Source: three-view drawing plus pictorial views. Frame: mm from the lowest corner of the part. A direction names the side the tool comes from. Coordinates: 2 decimals unless noted, no trailing zeros. Loops run counter-clockwise (first coordinate to the right, second up) from the corner with the lowest first, then second, coordinate; pieces in that order, holes last. Notation, with made-up numbers: M 34.5,78.5 L 60.5,78.5 A22 ccw 60.5,117.5 Z; hole C 28,-26 d6. An arc over 180 degrees is marked long. Use a Markdown table: item, result. Add a question column.
1. Section D-D on x = 7.75. Output: boundary loops of the cut face in (y, z).
2. Section A-A on y = 0.75. Output: boundary loops of the cut face in (x, z), then the cut area to 3 significant figures.
3. Line query: L1, parallel to X at y = 0.5, z = 8.5; L2, parallel to Z at x = 6.75, y = 1; L3, parallel to X at y = 1.15, z = 2.5. Output: solid intervals per line, ascending. Write a range as [from, to].
4. Section C-C on x = 6. Output: boundary loops of the cut face in (y, z), then the cut area to 3 significant figures.
5. Pin query (flat end, axial travel): pin 1 (6 mm diameter, centred on x = 5.5, z = 5.5, fed in from +Y); pin 2 (4 mm diameter, centred on y = 5.5, z = 4.5, fed in from +X). Return the tip coordinate at first contact, or that it passes through.
6. Section B-B on z = 8.5. Output: boundary loops of the cut face in (x, y), then the cut area to 3 significant figures.
7. Draft query along X for the marked faces 3, 4 and 5. Return one class per face: +X half, -X half, draft (parallel to the pull), parting line (faces both ways), or undercut.
8. Set-up query: the marked faces 1 and 2. Return all of +Z, -Z, +X, -X, +Y, -Y with unobstructed straight access to the full face (end or side cutting, diameter ignored); none if empty.
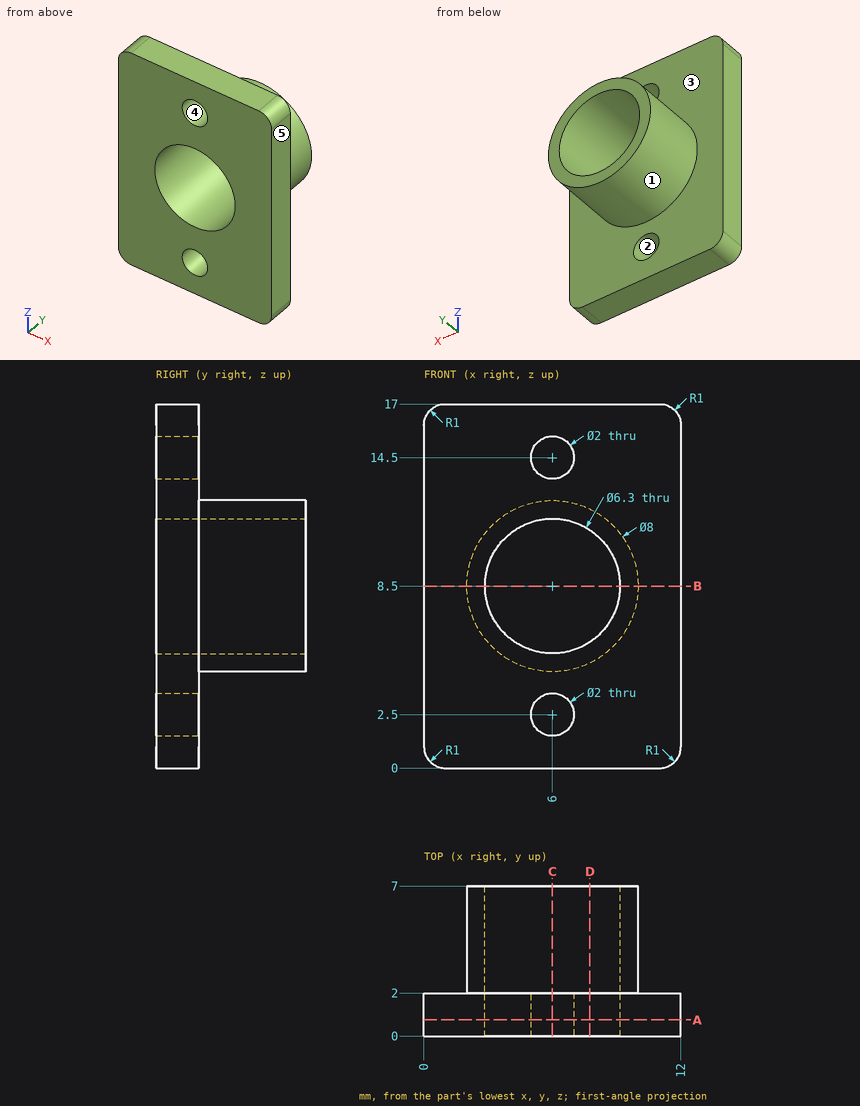
Answers below:
| question | item | result |
|---|---|---|
| 1 | outline | M 0,0 L 2,0 L 2,4.9 L 7,4.9 L 7,5.88 L 0,5.88 Z; M 0,11.12 L 7,11.12 L 7,12.1 L 2,12.1 L 2,17 L 0,17 Z |
| 2 | outline | M 0,1 A1 ccw 1,0 L 11,0 A1 ccw 12,1 L 12,16 A1 ccw 11,17 L 1,17 A1 ccw 0,16 Z; hole C 6,8.5 d6.3; hole C 6,2.5 d2; hole C 6,14.5 d2 |
| 2 | area | 166 mm² |
| 3 | L1 | x = [0, 2.85], [9.15, 12] |
| 3 | L2 | z = [0, 1.84], [3.16, 5.44], [11.56, 13.84], [15.16, 17] |
| 3 | L3 | x = [0, 5], [7, 12] |
| 4 | outline | M 0,0 L 2,0 L 2,1.5 L 0,1.5 Z; M 0,3.5 L 2,3.5 L 2,4.5 L 7,4.5 L 7,5.35 L 0,5.35 Z; M 0,11.65 L 7,11.65 L 7,12.5 L 2,12.5 L 2,13.5 L 0,13.5 Z; M 0,15.5 L 2,15.5 L 2,17 L 0,17 Z |
| 4 | area | 21.9 mm² |
| 5 | pin 1 | stops at y = 7 |
| 5 | pin 2 | stops at x = 9.46 |
| 6 | outline | M 0,0 L 2.85,0 L 2.85,7 L 2,7 L 2,2 L 0,2 Z; M 9.15,0 L 12,0 L 12,2 L 10,2 L 10,7 L 9.15,7 Z |
| 6 | area | 19.9 mm² |
| 7 | face 3 | draft |
| 7 | face 4 | undercut |
| 7 | face 5 | +X half |
| 8 | face 1 | +Y |
| 8 | face 2 | +Y, -Y |
